Design review of the part built by this model. Coordinates are the model's own, in mm. A direction names the side the tool comes from. Coordinates: 2 decimals unless noted, no trailing zeros. Loops run counter-clockwise (first coordinate to the right, second up) from the corner with the lowest first, then second, coordinate; pieces in that order, holes last. Notation, with made-up numbers: (63.25, -31) -> (77.25, -31) arc R17 ccw to (77.25, -11) -> close; hole circle Ø8 at (9, -5). An arc over 180 degrees is marked (long way). Answer in a Markdown table with one row per item.
```python
from build123d import *

# Parameters (mm, degrees)
SKETCH_1_R          = 87.5
EXTRUDE_1_DEPTH     = 18
SKETCH_2_R          = 72.5
EXTRUDE_2_DEPTH     = 10
SKETCH_3_R          = 50
EXTRUDE_3_DEPTH     = 8
SKETCH_4_R          = 60.5
SKETCH_4_R_2        = 51.5
CUT_EXTRUDE_1_DEPTH = 5
SKETCH_5_R          = 37.5
CUT_EXTRUDE_2_DEPTH = 129.873969443
CUT_EXTRUDE_2_DRAFT = 10


with BuildPart() as part:
    # 草图1 → 凸台-拉伸1 (new body)
    with BuildSketch(Plane.XY):
        Circle(SKETCH_1_R)
    extrude(amount=EXTRUDE_1_DEPTH)

    # 草图2 → 凸台-拉伸2 (add)
    with BuildSketch(Plane.XY.offset(18)):
        Circle(SKETCH_2_R)
    extrude(amount=EXTRUDE_2_DEPTH)

    # 草图3 → 凸台-拉伸3 (add)
    with BuildSketch(Plane.XY.offset(28)):
        Circle(SKETCH_3_R)
    extrude(amount=EXTRUDE_3_DEPTH)

    # 草图4 → 切除-拉伸1 (cut)
    with BuildSketch(Plane(origin=(0, 0, 0), x_dir=(-1, 0, 0), z_dir=(0, 0, -1))):
        Circle(SKETCH_4_R)
        Circle(SKETCH_4_R_2, mode=Mode.SUBTRACT)
    extrude(amount=-CUT_EXTRUDE_1_DEPTH, mode=Mode.SUBTRACT)


with BuildPart() as cut_extrude_2_tool:
    # 草图5 → 切除-拉伸2 (with draft: the straight prism first)
    with BuildSketch(Plane.XY.offset(36)):
        Circle(SKETCH_5_R)
    extrude(amount=-CUT_EXTRUDE_2_DEPTH)
    # 切除-拉伸2: the draft: its side faces are tilted about the plane it starts from
    cut_extrude_2_sides = [cut_extrude_2_tool.faces().sort_by_distance(p)[0] for p in [
        (-37.5, 0, -28.936984722),
    ]]
    draft(cut_extrude_2_sides, Plane.XY.offset(36), CUT_EXTRUDE_2_DRAFT)


with BuildPart() as part_1:
    add(part.part)

    # 切除-拉伸2: cut by cut_extrude_2_tool
    add(cut_extrude_2_tool.part, mode=Mode.SUBTRACT)


solid = part_1.part
```
(1) To check wall thickness, follow probe 1 along Y at (x, z) = (0, 1.25); probe 2 along Z at (x, y) = (65.5, -43); probe 3 along Y at (x, z) = (0, 3.25). State the ranges of each line that lie inside material, in increasing order.
Evaluation:
| item | result |
|---|---|
| probe 1 | y = -87.5 to -60.5, -51.5 to -43.63, 43.63 to 51.5, 60.5 to 87.5 |
| probe 2 | z = 0 to 18 |
| probe 3 | y = -87.5 to -60.5, -51.5 to -43.27, 43.27 to 51.5, 60.5 to 87.5 |
(2) For pin 1 (1 mm diameter, centred on x = 5.5, z = 5, fed in from -Y); pin 2 (1.5 mm diameter, centred on x = -50, z = 14, fed in from -Y); pin 3 (2 mm diameter, centred on x = 4.5, z = 30, fed in from +Y), all flat-tipped, find the tip position at first contact; note any pin that passes through.
Evaluation:
| item | result |
|---|---|
| pin 1 | stops at y = -87.36 |
| pin 2 | stops at y = -72.32 |
| pin 3 | stops at y = 49.88 |
(3) Take a section at C-C on y = -46.5. Give the boundary of the cut face in (x, z), and give its area (3 significant figures).
Evaluation:
| item | result |
|---|---|
| outline | (-74.12, 0) -> (-38.7, 0) -> (-38.7, 5) -> (-22.14, 5) -> (-22.14, 0) -> (22.14, 0) -> (22.14, 5) -> (38.7, 5) -> (38.7, 0) -> (74.12, 0) -> (74.12, 18) -> (55.62, 18) -> (55.62, 28) -> (18.38, 28) -> (18.38, 36) -> (-18.38, 36) -> (-18.38, 28) -> (-55.62, 28) -> (-55.62, 18) -> (-74.12, 18) -> close |
| area | 3,910 mm² |
(4) Take a section at A-A on x = 0. Give the boundary of the cut face in (y, z).
Evaluation:
| item | result |
|---|---|
| outline | (-87.5, 0) -> (-60.5, 0) -> (-60.5, 5) -> (-51.5, 5) -> (-51.5, 0) -> (-43.85, 0) -> (-37.5, 36) -> (-50, 36) -> (-50, 28) -> (-72.5, 28) -> (-72.5, 18) -> (-87.5, 18) -> close; (37.5, 36) -> (43.85, 0) -> (51.5, 0) -> (51.5, 5) -> (60.5, 5) -> (60.5, 0) -> (87.5, 0) -> (87.5, 18) -> (72.5, 18) -> (72.5, 28) -> (50, 28) -> (50, 36) -> close |
(5) Draft analysis for pull direction X (two halves, no side actions). For faces 4 (the cylindrical face through (47.69, 15.02, 31.94)), 5 (the flat face through (7, 37, 36)), 6 (the flat face through (-45, 27, 5)), state which applies: pulls with the +X half, pulls with the -X half, needs draft (parallel to the pull), parting line crosses it, or undercut.
Evaluation:
| item | result |
|---|---|
| face 4 | parting line crosses it |
| face 5 | needs draft |
| face 6 | undercut |
(6) Tool access review of faces 1 (the flat face through (-33, 65, 18)), 2 (the cylindrical face through (-64.49, 59.14, 8.87)), 3 (the cylindrical face through (13.12, -59.06, 2.46)): name each direction out of +Z, -Z, +X, -X, +Y, -Y from which nothing blocks a thin tool from reaching the whole face with its end or side.
Evaluation:
| item | result |
|---|---|
| face 1 | +Z |
| face 2 | +Z, -Z |
| face 3 | -Z |
(7) Take a section at D-D on z = 15.5. Give the boundary of the cut face in (x, y), and give its area (3 significant figures).
Evaluation:
| item | result |
|---|---|
| outline | circle Ø175 at (0, 0); hole circle Ø82.23 at (0, 0) |
| area | 18,700 mm² |
